For this review, take the finished solid that the model builds, in its own axes (mm). A direction names the side the tool comes from. Round coordinates to 2 decimals unless told otherwise and drop trailing zeros. Order: outer loops, then holes, each group sorted by start corner. A loop starts at its lowest first (then second) coordinate and runs counter-clockwise, first axis right, second up. Notation, with made-up numbers: M -14,86 L 19,86 A22 cw 19,111 Z; hole C 65,-9 d4. An arc over 180 degrees is marked long. Answer as a JSON object with one key per item and string values.
from build123d import *

# Parameters (mm, degrees)
SKETCH1_W                                        = 101.6
SKETCH1_H                                        = 50.8
BOSS_EXTRUDE1_DEPTH                              = 25.4
SKETCH2_R                                        = 11.1125
CUT_EXTRUDE1_DEPTH                               = 50.8
CBORE_FOR_1_2_SOCKET_HEAD_CAP_SCREW1_D           = 13.49248
CBORE_FOR_1_2_SOCKET_HEAD_CAP_SCREW1_DEPTH       = 50.8
CBORE_FOR_1_2_SOCKET_HEAD_CAP_SCREW1_CBORE_D     = 20.6375
CBORE_FOR_1_2_SOCKET_HEAD_CAP_SCREW1_CBORE_DEPTH = 12.7
CBORE_FOR_1_2_SOCKET_HEAD_CAP_SCREW1_TIP         = 4.053549943
SKETCH8_R                                        = 4.7625
CUT_EXTRUDE2_DEPTH                               = 117.397422652


with BuildPart() as part:
    # Sketch1 → Boss-Extrude1 (new body)
    with BuildSketch(Plane(origin=(0, 0, 0), x_dir=(0, 0, -1), z_dir=(1, 0, 0))):
        with Locations((50.8, 25.4)):
            Rectangle(SKETCH1_W, SKETCH1_H)
    extrude(amount=BOSS_EXTRUDE1_DEPTH)

    # Sketch2 → Cut-Extrude1 (cut)
    with BuildSketch(Plane(origin=(0, 50.8, 0), x_dir=(1, 0, 0), z_dir=(0, 1, 0))):
        with Locations(Location((12.7, 50.8, 0), (0, 0, 270))):
            Circle(SKETCH2_R)
    extrude(amount=-CUT_EXTRUDE1_DEPTH, mode=Mode.SUBTRACT)

    # CBORE for 1/2 Socket Head Cap Screw1
    with Locations(Plane(origin=(0, 50.8, 0), x_dir=(1, 0, 0), z_dir=(0, 1, 0))):
        with Locations((12.7, 88.9), (12.7, 12.7)):
            CounterBoreHole(CBORE_FOR_1_2_SOCKET_HEAD_CAP_SCREW1_D / 2, CBORE_FOR_1_2_SOCKET_HEAD_CAP_SCREW1_CBORE_D / 2, CBORE_FOR_1_2_SOCKET_HEAD_CAP_SCREW1_CBORE_DEPTH, depth=CBORE_FOR_1_2_SOCKET_HEAD_CAP_SCREW1_DEPTH)
            with Locations((0, 0, -(CBORE_FOR_1_2_SOCKET_HEAD_CAP_SCREW1_DEPTH + CBORE_FOR_1_2_SOCKET_HEAD_CAP_SCREW1_TIP / 2))):  # 118° drill point
                Cone(0, CBORE_FOR_1_2_SOCKET_HEAD_CAP_SCREW1_D / 2, CBORE_FOR_1_2_SOCKET_HEAD_CAP_SCREW1_TIP, mode=Mode.SUBTRACT)

    # Sketch8 → Cut-Extrude2 (cut, through all)
    with BuildSketch(Plane.ZY):
        with Locations((-50.8, 7.9375)):
            Circle(SKETCH8_R)
    extrude(amount=-CUT_EXTRUDE2_DEPTH, mode=Mode.SUBTRACT)


solid = part.part
1) Add section A-A on z = -12.7. State the section outline as (x, y) points, and give its area (3 significant figures).
Geometry check:
{"outline": "M 0,0 L 5.95,0 L 5.95,38.1 L 2.38,38.1 L 2.38,50.8 L 0,50.8 Z; M 19.45,0 L 25.4,0 L 25.4,50.8 L 23.02,50.8 L 23.02,38.1 L 19.45,38.1 Z", "area": "514 mm²"}
2) Machinability: for faces 5 (the cylindrical face through (9.073, 18.783, -18.388)), 6 (the flat face through (19.4, 38.1, -10.6)), which of the approach directions +Z, -Z, +X, -X, +Y, -Y give a long, thin tool a straight path to every point of the face, cutting with its end or side? Answer none if there is none.
Geometry check:
{"face 5": "+Y, -Y", "face 6": "+Y"}
3) Add section C-C on z = -50.8. State the section outline as (x, y) points (1 decimal), and give its area (3 significant figures).
Geometry check:
{"outline": "M 0,0 L 1.6,0 L 1.6,3.2 L 0,3.2 Z; M 0,12.7 L 1.6,12.7 L 1.6,50.8 L 0,50.8 Z; M 23.8,0 L 25.4,0 L 25.4,3.2 L 23.8,3.2 Z; M 23.8,12.7 L 25.4,12.7 L 25.4,50.8 L 23.8,50.8 Z", "area": "131 mm²"}
4) For L1, parallel to Z at x = 12.5, y = 17; L2, parallel to Z at x = 15.75, y = 21; L3, parallel to Y at x = 1.1, z = -50.8 (3 decimals), list the stretches that pass through material, from the lowest coordinate up.
Geometry check:
{"L1": "z = -101.6 to -95.64, -82.16 to -61.91, -39.69 to -19.44, -5.96 to 0", "L2": "z = -101.6 to -94.92, -82.88 to -61.49, -40.11 to -18.72, -6.68 to 0", "L3": "y = 0 to 3.175, 12.7 to 50.8"}
5) Add section D-D on y = 41.5. State the section outline as (x, z) points (1 decimal).
Geometry check:
{"outline": "M 0,-101.6 L 25.4,-101.6 L 25.4,0 L 0,0 Z; hole C 12.7,-50.8 d22.2; hole C 12.7,-88.9 d20.6; hole C 12.7,-12.7 d20.6"}
6) Add section B-B on x = 12.7. State the section outline as (y, z) points, and give its area (3 significant figures).
Geometry check:
{"outline": "M 0,-101.6 L 50.8,-101.6 L 50.8,-99.22 L 38.1,-99.22 L 38.1,-95.65 L 0,-95.65 Z; M 0,-82.15 L 38.1,-82.15 L 38.1,-78.58 L 50.8,-78.58 L 50.8,-61.91 L 0,-61.91 Z; M 0,-39.69 L 50.8,-39.69 L 50.8,-23.02 L 38.1,-23.02 L 38.1,-19.45 L 0,-19.45 Z; M 0,-5.95 L 38.1,-5.95 L 38.1,-2.38 L 50.8,-2.38 L 50.8,0 L 0,0 Z", "area": "2,480 mm²"}
7) Mouldability with a two-part tool opening along Z and no side actions: class faces 1 (the flat face through (13, 0, -39)), 2 (the flat face through (15, 38.1, -82)), 3 (the flat face through (13, 25, -101.6)), 4 (the flat face through (13, 25, 0)) as +Z half, -Z half, draft (parallel to the pull), parting line (faces both ways), or undercut.
Geometry check:
{"face 1": "draft", "face 2": "undercut", "face 3": "-Z half", "face 4": "+Z half"}
